Verification items for the finished model (mm, model axes). Give positions to 0.01 mm unless a question says otherwise; leave off trailing zeros. Write each loop counter-clockwise with the first axis right and the second up, starting at its lowest first coordinate (ties: lowest second). Pieces come first, ordered by that corner, then holes. Notation, with made-up numbers: (15.25, 4) -> (24.25, 4) arc R29 ccw to (24.25, 38) -> close; hole circle Ø2 at (-13, 0.5). An arc over 180 degrees is marked (long way). Use one line per item in the form item = value. Start each with the question number.
(1) Scan lines: L1, parallel to X at y = -4.5, z = -26.5; L2, parallel to Z at x = 39.5, y = -5; L3, parallel to X at y = -5.5, z = 34. Record each from-to range of solid material in increasing order.
(2) Depth check by flat-ended pin: pin 1 Ø4 at (x, y) = (21, -1.5) entering from +Z; pin 2 Ø3 at (x, z) = (7.5, -29.5) entering from +Y; pin 3 Ø4 at (x, y) = (10, -1) entering from -Z; pin 4 Ø2 at (y, z) = (-3, 31) entering from -X. Enter the tip coordinate at first touch or a pass-through.
(3) Section check A-A, the plane z = -29.5. Record the cut outline in (x, y), plus the area to 3 significant figures.
(4) Release check for a two-part mould opening along Z. For faces 1 (the face through (32.156, -3.431, 13.53)), 2 (the face through (5.076, -3.431, 9.759)), 3 (the face through (28.114, -3.431, 21.148)), 4 (the face through (-11, 0, 9)) record: pulls with the +Z half, pulls with the -Z half, needs draft (parallel to the pull), parting line crosses it, or undercut.
from build123d import *

# Parameters (mm, degrees)
F1_DEPTH = 6.96


# Not quite as in the source:
# - a feature of the source that left no trace in its solid (it failed there, or was rolled back) is left out
# - a feature names something its author has since deleted; it is built from what else it names


with BuildPart() as f1:
    # F0 (on Front) → F1 (new body)
    with BuildSketch(Plane.XZ):
        with BuildLine():
            Line((-4.9618439889, 30.8489073878), (-10.120921757, 36.7311440441))
            ThreePointArc((-10.120921757, 36.7311440441), (-12.9466687362, 35.832858784), (-15.6940034453, 34.7175496811))
            Line((-15.6940034453, 34.7175496811), (-15.6940034453, 27.0180169266))
            ThreePointArc((-15.6940034453, 27.0180169266), (-10.5040439231, 29.4268592285), (-4.9618439889, 30.8489073878))
        make_face()
        with BuildLine():
            ThreePointArc((-15.6940034453, 34.7175496811), (-12.9466687362, 35.832858784), (-10.120921757, 36.7311440441))
            Line((-10.120921757, 36.7311440441), (-15.6940034453, 43.0854164294))
            Line((-15.6940034453, 43.0854164294), (-15.6940034453, 34.7175496811))
        make_face()
        with BuildLine():
            Line((0.3367577987, 24.8075893339), (-4.9618439889, 30.8489073878))
            ThreePointArc((-4.9618439889, 30.8489073878), (-10.5040439231, 29.4268592285), (-15.6940034453, 27.0180169266))
            Line((-15.6940034453, 27.0180169266), (-15.6940034453, 18.6877066835))
            Line((-15.6940034453, 18.6877066835), (-6.1980460207, 17.0157598588))
            Line((-6.1980460207, 17.0157598588), (0.3367577987, 24.8075893339))
        make_face()
        with BuildLine():
            Line((5.349116457, 30.7841182417), (0.3367577987, 24.8075893339))
            Line((0.3367577987, 24.8075893339), (-6.1980460207, 17.0157598588))
            Line((-6.1980460207, 17.0157598588), (-15.6940034453, 18.6877066835))
            Line((-15.6940034453, 18.6877066835), (-15.6940034453, 10.6181583146))
            Line((-15.6940034453, 10.6181583146), (-25.0790561702, 4.6957263488))
            Line((-25.0790561702, 4.6957263488), (-18.6598426779, -3.2950419376))
            Line((-18.6598426779, -3.2950419376), (-21.8185465433, -12.6017368372))
            Line((-21.8185465433, -12.6017368372), (-12.1835113634, -14.5123768209))
            Line((-12.1835113634, -14.5123768209), (-8.6159947437, -23.6812639315))
            Line((-8.6159947437, -23.6812639315), (0, -18.9485363587))
            Line((0, -18.9485363587), (8.6238023794, -23.6784231328))
            Line((8.6238023794, -23.6784231328), (12.1835113634, -14.5123768209))
            Line((12.1835113634, -14.5123768209), (21.8258896669, -12.5939120432))
            Line((21.8258896669, -12.5939120432), (18.6614871852, -3.2857154732))
            Line((18.6614871852, -3.2857154732), (24.8148121143, 4.3819151105))
            Line((24.8148121143, 4.3819151105), (29.5186280009, 10.2433189804))
            Line((29.5186280009, 10.2433189804), (34.4156358122, 16.3454584408))
            Line((34.4156358122, 16.3454584408), (39.7056170429, 22.9372803158))
            Line((39.7056170429, 22.9372803158), (16.1926081875, 19.3073954844))
            Line((16.1926081875, 19.3073954844), (15.85724841, 34.6432918884))
            ThreePointArc((15.85724841, 34.6432918884), (14.4513233415, 35.2529325543), (13.0220201926, 35.8055441252))
            Line((13.0220201926, 35.8055441252), (10.6792184181, 29.3637408511))
            ThreePointArc((10.6792184181, 29.3637408511), (8.0455731741, 30.1917825756), (5.349116457, 30.7841182417))
        make_face()
        with BuildLine():
            ThreePointArc((3.7596383758, 10.3375586713), (9.0098840762, 6.3104666177), (11, 0))
            ThreePointArc((11, 0), (-9.0098840762, -6.3104666177), (3.7596383758, 10.3375586713))
        make_face(mode=Mode.SUBTRACT)
        with BuildLine():
            Line((-15.6940034453, 10.6181583146), (-15.6940034453, 18.6877066835))
            Line((-15.6940034453, 18.6877066835), (-23.8953753875, 20.1317167147))
            ThreePointArc((-23.8953753875, 20.1317167147), (-27.1646586752, 15.4387921111), (-29.52374385, 10.2285645068))
            Line((-29.52374385, 10.2285645068), (-25.0790561702, 4.6957263488))
            Line((-25.0790561702, 4.6957263488), (-15.6940034453, 10.6181583146))
        make_face()
        with BuildLine():
            Line((10.2959158336, 36.6824769767), (5.349116457, 30.7841182417))
            ThreePointArc((5.349116457, 30.7841182417), (8.0455731741, 30.1917825756), (10.6792184181, 29.3637408511))
            Line((10.6792184181, 29.3637408511), (13.0220201926, 35.8055441252))
            ThreePointArc((13.0220201926, 35.8055441252), (11.6672099465, 36.2696320916), (10.2959158336, 36.6824769767))
        make_face()
        with BuildLine():
            ThreePointArc((-29.52374385, 10.2285645068), (-27.1646586752, 15.4387921111), (-23.8953753875, 20.1317167147))
            Line((-23.8953753875, 20.1317167147), (-31.476903581, 21.4665912747))
            Line((-31.476903581, 21.4665912747), (-39.7170759686, 22.9174328742))
            Line((-39.7170759686, 22.9174328742), (-29.52374385, 10.2285645068))
        make_face()
        with BuildLine():
            Line((15.6724677094, 43.0932547963), (10.2959158336, 36.6824769767))
            ThreePointArc((10.2959158336, 36.6824769767), (11.6672099465, 36.2696320916), (13.0220201926, 35.8055441252))
            Line((13.0220201926, 35.8055441252), (15.6724677094, 43.0932547963))
        make_face()
        with BuildLine():
            Line((-18.6598426779, -3.2950419376), (-25.0790561702, 4.6957263488))
            Line((-25.0790561702, 4.6957263488), (-31.2348698324, 0.8111037816))
            ThreePointArc((-31.2348698324, 0.8111037816), (-30.7987467244, -5.2642362214), (-29.1922235992, -11.139527105))
            Line((-29.1922235992, -11.139527105), (-21.8185465433, -12.6017368372))
            Line((-21.8185465433, -12.6017368372), (-18.6598426779, -3.2950419376))
        make_face()
        with BuildLine():
            Line((15.85724841, 34.6432918884), (15.6724677094, 43.0932547963))
            Line((15.6724677094, 43.0932547963), (13.0220201926, 35.8055441252))
            ThreePointArc((13.0220201926, 35.8055441252), (14.4513233415, 35.2529325543), (15.85724841, 34.6432918884))
        make_face()
        with BuildLine():
            ThreePointArc((-29.1922235992, -11.139527105), (-30.7987467244, -5.2642362214), (-31.2348698324, 0.8111037816))
            Line((-31.2348698324, 0.8111037816), (-37.9458459601, -3.4238537307))
            ThreePointArc((-37.9458459601, -3.4238537307), (-37.5339500378, -6.54313339), (-36.8660833418, -9.6177907563))
            Line((-36.8660833418, -9.6177907563), (-29.1922235992, -11.139527105))
        make_face()
        with BuildLine():
            Line((-12.1835113634, -14.5123768209), (-21.8185465433, -12.6017368372))
            Line((-21.8185465433, -12.6017368372), (-24.2350154824, -19.7215366379))
            ThreePointArc((-24.2350154824, -19.7215366379), (-20.078672611, -23.9399642642), (-15.2010519849, -27.2984065715))
            Line((-15.2010519849, -27.2984065715), (-8.6159947437, -23.6812639315))
            Line((-8.6159947437, -23.6812639315), (-12.1835113634, -14.5123768209))
        make_face()
        with BuildLine():
            ThreePointArc((-36.8660833418, -9.6177907563), (-37.5339500378, -6.54313339), (-37.9458459601, -3.4238537307))
            Line((-37.9458459601, -3.4238537307), (-45.15608724, -7.9738722218))
            Line((-45.15608724, -7.9738722218), (-36.8660833418, -9.6177907563))
        make_face()
        with BuildLine():
            ThreePointArc((-15.2010519849, -27.2984065715), (-20.078672611, -23.9399642642), (-24.2350154824, -19.7215366379))
            Line((-24.2350154824, -19.7215366379), (-26.7496429738, -27.1305473733))
            ThreePointArc((-26.7496429738, -27.1305473733), (-24.4831574997, -29.1922078446), (-22.0583421712, -31.0650855569))
            Line((-22.0583421712, -31.0650855569), (-15.2010519849, -27.2984065715))
        make_face()
        with BuildLine():
            ThreePointArc((-22.0583421712, -31.0650855569), (-24.4831574997, -29.1922078446), (-26.7496429738, -27.1305473733))
            Line((-26.7496429738, -27.1305473733), (-29.4660634378, -35.1341138854))
            Line((-29.4660634378, -35.1341138854), (-22.0583421712, -31.0650855569))
        make_face()
        with BuildLine():
            Line((0, -18.9485363587), (-8.6159947437, -23.6812639315))
            Line((-8.6159947437, -23.6812639315), (-5.8908957162, -30.6850506021))
            ThreePointArc((-5.8908957162, -30.6850506021), (0.0065066962, -31.2453987085), (5.9036752179, -30.6825944423))
            Line((5.9036752179, -30.6825944423), (8.6238023794, -23.6784231328))
            Line((8.6238023794, -23.6784231328), (0, -18.9485363587))
        make_face()
        with BuildLine():
            ThreePointArc((5.9036752179, -30.6825944423), (0.0065066962, -31.2453987085), (-5.8908957162, -30.6850506021))
            Line((-5.8908957162, -30.6850506021), (-3.0535035766, -37.9774421981))
            Line((-3.0535035766, -37.9774421981), (0.0114589257, -45.8547131899))
            Line((0.0114589257, -45.8547131899), (5.9036752179, -30.6825944423))
        make_face()
        with BuildLine():
            Line((12.1835113634, -14.5123768209), (8.6238023794, -23.6784231328))
            Line((8.6238023794, -23.6784231328), (15.2124188317, -27.2920738691))
            ThreePointArc((15.2124188317, -27.2920738691), (20.0896378001, -23.930763378), (24.2448691352, -19.7094216914))
            Line((24.2448691352, -19.7094216914), (21.8258896669, -12.5939120432))
            Line((21.8258896669, -12.5939120432), (12.1835113634, -14.5123768209))
        make_face()
        with BuildLine():
            Line((31.2416193325, 0.4860085148), (24.8148121143, 4.3819151105))
            Line((24.8148121143, 4.3819151105), (18.6614871852, -3.2857154732))
            Line((18.6614871852, -3.2857154732), (21.8258896669, -12.5939120432))
            Line((21.8258896669, -12.5939120432), (29.1968594713, -11.1273707499))
            ThreePointArc((29.1968594713, -11.1273707499), (30.7720664648, -5.418017006), (31.2416193325, 0.4860085148))
        make_face()
        with BuildLine():
            ThreePointArc((24.2448691352, -19.7094216914), (20.0896378001, -23.930763378), (15.2124188317, -27.2920738691))
            Line((15.2124188317, -27.2920738691), (22.0728280834, -31.0547944833))
            ThreePointArc((22.0728280834, -31.0547944833), (24.4972570827, -29.1803768897), (26.7631992818, -27.117174709))
            Line((26.7631992818, -27.117174709), (24.2448691352, -19.7094216914))
        make_face()
        with BuildLine():
            Line((37.9323840026, -3.569908105), (31.2416193325, 0.4860085148))
            ThreePointArc((31.2416193325, 0.4860085148), (30.7720664648, -5.418017006), (29.1968594713, -11.1273707499))
            Line((29.1968594713, -11.1273707499), (36.8705647308, -9.6005966708))
            ThreePointArc((36.8705647308, -9.6005966708), (37.5228275313, -6.6066189578), (37.9323840026, -3.569908105))
        make_face()
        with BuildLine():
            ThreePointArc((26.7631992818, -27.117174709), (24.4972570827, -29.1803768897), (22.0728280834, -31.0547944833))
            Line((22.0728280834, -31.0547944833), (29.4836195306, -35.1193825745))
            Line((29.4836195306, -35.1193825745), (26.7631992818, -27.117174709))
        make_face()
        with BuildLine():
            Line((45.1600668832, -7.951302544), (37.9323840026, -3.569908105))
            ThreePointArc((37.9323840026, -3.569908105), (37.5228275313, -6.6066189578), (36.8705647308, -9.6005966708))
            Line((36.8705647308, -9.6005966708), (45.1600668832, -7.951302544))
        make_face()
    extrude(amount=F1_DEPTH)


solid = f1.part
Completed:
q1.L1 = -26.54 to -13.75, -7.52 to 7.53, 13.77 to 26.55
q1.L2 = -9.08 to -4.52, 22.68 to 22.91
q1.L3 = -15.69 to -7.73, 8.05 to 15.87
q2.pin_1 = 20.36
q2.pin_2 = 0
q2.pin_3 = -25.53
q2.pin_4 = -15.69
q3.outline = (-27.55, -6.96) -> (-19.21, -6.96) -> (-19.21, 0) -> (-27.55, 0) -> close; (-6.35, -6.96) -> (6.36, -6.96) -> (6.36, 0) -> (-6.35, 0) -> close; (19.24, -6.96) -> (27.57, -6.96) -> (27.57, 0) -> (19.24, 0) -> close
q3.area = 205 mm²
q4.face_1 = undercut
q4.face_2 = undercut
q4.face_3 = pulls with the +Z half
q4.face_4 = needs draft
